Check sheet for the drawn part. Datum: minimum x, y, z corner. Units: mm. Coordinates: 2 decimals unless noted, no trailing zeros. Order: outer loops, then holes, each group sorted by start corner. A loop starts at its lowest first (then second) coordinate and runs counter-clockwise, first axis right, second up. Notation, with made-up numbers: M 4.5,45 L 48.5,45 A19 ccw 48.5,61 Z; hole C -16.5,36.5 d8. An arc over 180 degrees is marked long. Return JSON: item names as keys, results as strings. Group by question number.
Q1. Section check B-B, the plane x = 3.75. Enter the section's corners in (y, z) (1 decimal).
Q2. Section check C-C, the plane y = 64. Enter the section's corners in (x, z) (1 decimal).
Q3. Mould release check, pull along Z, two halves, no side actions. Record for the marked faces 1, 2, 3 and 4: pulls with the +Z half, pulls with the -Z half, needs draft (parallel to the pull), parting line crosses it, or undercut.
Q4. Section check D-D, the plane y = 53. Enter the section's corners in (x, z), then the cut area to 3 significant figures.
Q5. Section check A-A, the plane z = 22.5. Enter the section's corners in (x, y).
Q6. Go/stop test with flat-tipped pins: pin 1 Ø1 at (x, y) = (3.5, 27.5) entering from -Z; pin 2 Ø1.5 at (x, z) = (2.5, 26) entering from +Y (1 decimal); pin 3 Ø2 at (x, y) = (2, 38.5) entering from +Z. Record where each tip stops, or that it passes through.
Q7. Thickness scan on probe 1 along Y at (x, z) = (2.15, 22.5); probe 2 along Y at (x, z) = (3.65, 20.5); probe 3 along X at (y, z) = (16, 40). Record the ranges inside material, lowest first.
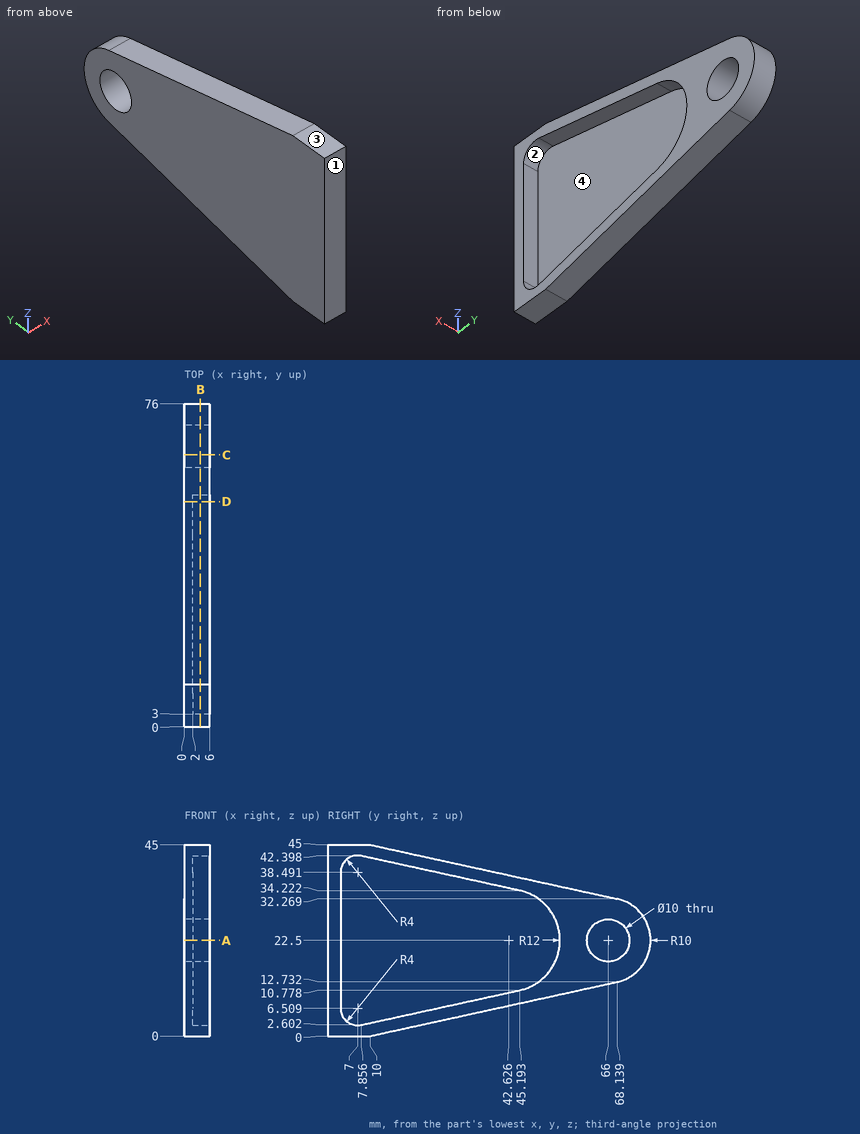
Numbers:
{
 "1": {"outline": "M 0,0 L 10,0 L 68.1,12.7 A10 ccw 68.1,32.3 L 10,45 L 0,45 Z; hole M 3,6.5 A4 ccw 7.9,2.6 L 45.2,10.8 A12 ccw 45.2,34.2 L 7.9,42.4 A4 ccw 3,38.5 Z; hole C 66,22.5 d10"},
 "2": {"outline": "M 0,11.8 L 6,11.8 L 6,17.9 L 0,17.9 Z; M 0,27.1 L 6,27.1 L 6,33.2 L 0,33.2 Z"},
 "3": {"face 1": "needs draft", "face 2": "undercut", "face 3": "pulls with the +Z half", "face 4": "undercut"},
 "4": {"outline": "M 0,9.42 L 6,9.42 L 6,16.47 L 2,16.47 L 2,28.53 L 6,28.53 L 6,35.58 L 0,35.58 Z", "area": "109 mm2"},
 "5": {"outline": "M 0,0 L 6,0 L 6,3 L 2,3 L 2,54.63 L 6,54.63 L 6,61 L 0,61 Z; M 0,71 L 6,71 L 6,76 L 0,76 Z"},
 "6": {"pin 1": "stops at z = 3.72", "pin 2": "stops at y = 75.6", "pin 3": "stops at z = 38.98"},
 "7": {"probe 1": "y = 0 to 3, 54.63 to 61, 71 to 76", "probe 2": "y = 0 to 3, 54.46 to 61.42, 70.58 to 75.8", "probe 3": "x = 0 to 2"}
}
